```python
from build123d import *

# Parameters (mm, degrees)
BOSS_EXTRUDE1_DEPTH       = 8.55
SKETCH1_4_W               = 18
SKETCH1_4_H               = 23.4
BOSS_EXTRUDE2_DEPTH       = 2
SKETCH2_W                 = 20.04
SKETCH2_H                 = 24.05
CUT_EXTRUDE1_DEPTH        = 3.55
SKETCH3_W                 = 6
SKETCH3_H                 = 3
BOSS_EXTRUDE4_DEPTH       = 2
FILLET1_R                 = 2
BOSS_EXTRUDE5_DEPTH       = 23.5
SKETCH6_W                 = 2
SKETCH6_H                 = 3.111945503
SKETCH6_W_2               = 9.5
CUT_EXTRUDE2_DEPTH        = 23
SKETCH7_W                 = 5
SKETCH7_H                 = 1.291023664
BOSS_EXTRUDE6_DEPTH       = 1
BOSS_EXTRUDE11_DEPTH      = 2
BOSS_EXTRUDE11_DEPTH_BACK = 15
SKETCH8_R                 = 3
CUT_EXTRUDE3_DEPTH        = 2
CUT_EXTRUDE3_DEPTH_BACK   = 15
SKETCH8_5_R               = 1.5
SKETCH10_R                = 4
BOSS_EXTRUDE13_DEPTH      = 2.5


with BuildPart() as part:
    # Sketch1 → Boss-Extrude1 (new body)
    with BuildSketch(Plane(origin=(0, 0, 0), x_dir=(1, 0, 0), z_dir=(0, 1, 0))):
        Polygon((-11.75, 13), (-11.75, -13), (-9, -13), (-9, 10.4), (9, 10.4), (9, -13), (11.75, -13), (11.75, 13), align=None)
    extrude(amount=BOSS_EXTRUDE1_DEPTH)

    # Sketch1_4 → Boss-Extrude2 (add)
    with BuildSketch(Plane(origin=(0, 0, 0), x_dir=(1, 0, 0), z_dir=(0, 1, 0))):
        with Locations((0, -1.3)):
            Rectangle(SKETCH1_4_W, SKETCH1_4_H)
    extrude(amount=BOSS_EXTRUDE2_DEPTH)

    # Sketch2 → Cut-Extrude1 (cut)
    with BuildSketch(Plane(origin=(0, 8.55, 0), x_dir=(1, 0, 0), z_dir=(0, 1, 0))):
        with Locations((0, -0.975)):
            Rectangle(SKETCH2_W, SKETCH2_H)
    extrude(amount=-CUT_EXTRUDE1_DEPTH, mode=Mode.SUBTRACT)

    # Sketch3 → Boss-Extrude4 (add)
    with BuildSketch(Plane.XY.offset(13)):
        Polygon((-11.75, 8.55), (-3, 8.55), (3, 8.55), (11.75, 8.55), (11.75, 0), (3, 0), (-3, 0), (-11.75, 0), align=None)
        with Locations((0, 3.5)):
            Rectangle(SKETCH3_W, SKETCH3_H, mode=Mode.SUBTRACT)
    extrude(amount=-BOSS_EXTRUDE4_DEPTH)

    # Fillet1
    fillet1_edges = [part.edges().sort_by_distance(p)[0] for p in [
        (-11.75, 4.275, 13),
        (-11.75, 4.275, -13),
        (11.75, 4.275, -13),
        (11.75, 4.275, 13),
    ]]
    fillet(fillet1_edges, radius=FILLET1_R)

    # Sketch5 → Boss-Extrude5 (add)
    with BuildSketch(Plane(origin=(11.75, 0, 0), x_dir=(0, 0, -1), z_dir=(1, 0, 0))):
        Polygon((-13, 0), (-16.111945503, 8.55), (-13, 8.55), align=None)
    extrude(amount=-BOSS_EXTRUDE5_DEPTH)

    # Sketch6 → Cut-Extrude2 (cut)
    with BuildSketch(Plane(origin=(0, 8.55, 0), x_dir=(1, 0, 0), z_dir=(0, 1, 0))):
        with Locations((-10.75, -14.555972752)):
            Rectangle(SKETCH6_W, SKETCH6_H)
        with Locations((10.75, -14.555972752)):
            Rectangle(SKETCH6_W, SKETCH6_H)
        with Locations((0, -14.555972752)):
            Rectangle(SKETCH6_W_2, SKETCH6_H)
    extrude(amount=-CUT_EXTRUDE2_DEPTH, mode=Mode.SUBTRACT)

    # Sketch7 → Boss-Extrude6 (add)
    with BuildSketch(Plane(origin=(0, -4.178119463, 11.47928888), x_dir=(1, 0, 0), z_dir=(0, -0.34202014332566966, 0.939692620785908))):
        with Locations((7.25, 12.899469986)):
            Rectangle(SKETCH7_W, SKETCH7_H)
    extrude(amount=BOSS_EXTRUDE6_DEPTH)

    # Sketch8 → Boss-Extrude11 (add, two sides: drawn at the far end of the back side and taken through both)
    with BuildSketch(Plane(origin=(0, 12.728119463, 4.632656623), x_dir=(1, 0, 0), z_dir=(0, 0.939692620785908, 0.3420201433256697)).offset(-BOSS_EXTRUDE11_DEPTH_BACK)):
        with Locations(Location((7.25, -13.71600407, 0), (0, 0, 270))):
            Circle(SKETCH8_R)
        with Locations(Location((-7.25, -13.71600407, 0), (0, 0, 270))):
            Circle(SKETCH8_R)
    extrude(amount=BOSS_EXTRUDE11_DEPTH + BOSS_EXTRUDE11_DEPTH_BACK)

    # Sketch8_5 → Cut-Extrude3 (cut, two sides: drawn at the far end of the back side and taken through both)
    with BuildSketch(Plane(origin=(0, 12.728119463, 4.632656623), x_dir=(1, 0, 0), z_dir=(0, 0.939692620785908, 0.3420201433256697)).offset(-CUT_EXTRUDE3_DEPTH_BACK)):
        with Locations(Location((-7.25, -13.71600407, 0), (0, 0, 270))):
            Circle(SKETCH8_5_R)
        with BuildLine():
            ThreePointArc((5.835786438, -13.21600407), (6.996347032, -15.19440191), (8.75, -13.71600407))
            ThreePointArc((8.75, -13.71600407), (8.728397839, -13.462351102), (8.664213562, -13.21600407))
            Line((8.664213562, -13.21600407), (5.835786438, -13.21600407))
        make_face()
        with BuildLine():
            Line((5.835786438, -13.21600407), (8.664213562, -13.21600407))
            ThreePointArc((8.664213562, -13.21600407), (7.25, -12.21600407), (5.835786438, -13.21600407))
        make_face()
    extrude(amount=CUT_EXTRUDE3_DEPTH + CUT_EXTRUDE3_DEPTH_BACK, mode=Mode.SUBTRACT)

    # Sketch10 → Boss-Extrude13 (add)
    with BuildSketch(Plane(origin=(0, 8.55, 0), x_dir=(1, 0, 0), z_dir=(0, 1, 0))):
        with BuildLine():
            Line((-5.75, -11), (5.75, -11))
            Line((5.75, -11), (5.75, -17.5))
            ThreePointArc((5.75, -17.5), (4.285533906, -21.035533906), (0.75, -22.5))
            Line((0.75, -22.5), (-0.75, -22.5))
            ThreePointArc((-0.75, -22.5), (-4.285533906, -21.035533906), (-5.75, -17.5))
            Line((-5.75, -17.5), (-5.75, -11))
        make_face()
        with Locations(Location((0, -17.1, 0), (0, 0, 270))):
            Circle(SKETCH10_R, mode=Mode.SUBTRACT)
    extrude(amount=-BOSS_EXTRUDE13_DEPTH)


solid = part.part
```
Geometry check sheet. Reference: the model listing, model coordinates, mm. A direction names the side the tool comes from. Round coordinates to 2 decimals unless told otherwise and drop trailing zeros. Loops run counter-clockwise (first coordinate to the right, second up) from the corner with the lowest first, then second, coordinate; pieces in that order, holes last. Notation, with made-up numbers: (-26.5, 39.5) - (-10.5, 39.5) arc R14 cw to (-10.5, 47.5) - close; hole circle Ø2 at (51, -26). An arc over 180 degrees is marked (long way). Write item = value, one per line. Start each with the question number.
1. Section check D-D on y = 7. Give the number of separate pieces and of enclosed holes in the cut face, then the cut area to 3 significant figures.
2. Section check A-A on x = 0. Enter the section's corners in (y, z), then the cut area to 3 significant figures.
3. Depth check by flat-ended pin: pin 1 (0.9 mm diameter, centred on y = 4, z = 14.5, fed in from +X); pin 2 (2 mm diameter, centred on y = 3, z = 12, fed in from -X); pin 3 (6 mm diameter, centred on x = 0.5, z = -0.5, fed in from +Y); pin 4 (1.8 mm diameter, centred on x = 1, y = 3.5, fed in from +Z). Enter the tip coordinate at first touch or a pass-through.
4. Section check B-B on z = -9.5. Enter the section's corners in (x, y).
5. Section check C-C on x = -3.5. Enter the section's corners in (y, z).
6. Set-up check for faces 5 (the face through (-4.75, 5, 14)), 6 (the face through (9.75, 6, 14)), 7 (the face through (3, 3, 12)): record each of +Z, -Z, +X, -X, +Y, -Y from which the full face is reachable in a straight line by a thin tool's end or side.
7. Mould release check, pull along Z, two halves, no side actions. Record for faces 1 (the face through (-8.58, 1.58, 15.91)), 2 (the face through (0, 5, 12)), 3 (the face through (-11.15, 4.33, -12.43)), 4 (the face through (-9.75, 6, 14)): released by +Z, released by -Z, zero draft, split by the parting line, or undercut.
8. Thickness scan on line 1 (X direction, y = 6.7, z = 17.1); line 2 (X direction, y = 2.25, z = 9.5); line 3 (Z direction, x = 6, y = -2.25). Record the ranges inside material, lowest first.
Working result:
q1.separate_pieces = 1
q1.enclosed_holes = 4
q1.area = 258 mm^2
q2.outline = (0, -13) - (8.55, -13) - (8.55, -11.05) - (5, -11.05) - (5, -10.4) - (2, -10.4) - (2, 13) - (0, 13) - close; (5, 11) - (8.55, 11) - (8.55, 13.1) - (6.05, 13.1) - (6.05, 13) - (5, 13) - close; (6.05, 21.1) - (8.55, 21.1) - (8.55, 22.5) - (6.05, 22.5) - close
q2.area = 77.6 mm^2
q3.pin_1 = 10.08
q3.pin_2 = -11.75
q3.pin_3 = 2
q3.pin_4 = -10.4
q4.outline = (-11.75, 0) - (11.75, 0) - (11.75, 8.55) - (10.02, 8.55) - (10.02, 5) - (9, 5) - (9, 2) - (-9, 2) - (-9, 5) - (-10.02, 5) - (-10.02, 8.55) - (-11.75, 8.55) - close
q5.outline = (0, -13) - (8.55, -13) - (8.55, -11.05) - (5, -11.05) - (5, -10.4) - (2, -10.4) - (2, 11) - (8.55, 11) - (8.55, 15.16) - (6.05, 15.16) - (6.05, 13) - (0, 13) - close; (6.05, 19.04) - (8.55, 19.04) - (8.55, 21.68) - (6.05, 21.68) - close
q6.face_5 = none
q6.face_6 = +X, +Y
q6.face_7 = +Z
q7.face_1 = undercut
q7.face_2 = zero draft
q7.face_3 = released by -Z
q7.face_4 = undercut
q8.line_1 = -10.25 to -8.75, -5.75 to -4, 4 to 5.75, 8.75 to 10.25
q8.line_2 = -11.75 to -9, 9 to 11.75
q8.line_3 = 10.88 to 12.89, 14.66 to 16.68
